from build123d import *

# Parameters (mm, degrees)
EXTRUDE_1_DEPTH          = 10
HOLE_WIZARD_M1_6_1_D     = 1.25
HOLE_WIZARD_M1_6_1_DEPTH = 4.95
HOLE_WIZARD_M1_6_1_TIP   = 0.375537887


with BuildPart() as part:
    # 草图2 → 凸台-拉伸1 (new body)
    with BuildSketch(Plane(origin=(0, 0, 0), x_dir=(1, 0, 0), z_dir=(0, 1, 0))):
        Polygon((7, 11), (-7, 11), (-7, 1), (-10, 1), (-10, 0), (-6, 0), (-6, 10), (6, 10), (6, 0), (10, 0), (10, 1), (7, 1), align=None)
    extrude(amount=EXTRUDE_1_DEPTH)

    # M1.6 螺纹孔1
    with Locations(Plane(origin=(0, 0, -1), x_dir=(-1, 0, 0), z_dir=(0, 0, -1))):
        with Locations((-8.5, 8), (8.5, 8), (8.5, 2), (-8.5, 2)):
            Hole(HOLE_WIZARD_M1_6_1_D / 2, depth=HOLE_WIZARD_M1_6_1_DEPTH)
            with Locations((0, 0, -(HOLE_WIZARD_M1_6_1_DEPTH + HOLE_WIZARD_M1_6_1_TIP / 2))):  # 118° drill point
                Cone(0, HOLE_WIZARD_M1_6_1_D / 2, HOLE_WIZARD_M1_6_1_TIP, mode=Mode.SUBTRACT)


solid = part.part
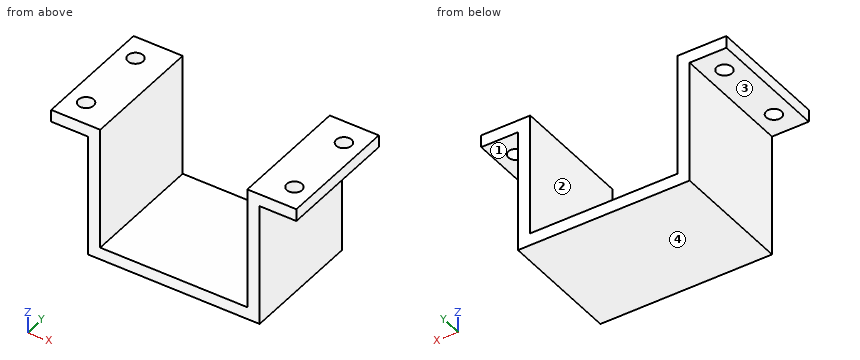
Read the model definition and answer for the solid it produces. Units are mm, in the model's axes. Face numbers are marked on the shaded views. A direction names the side the tool comes from. Round coordinates to 2 decimals unless told otherwise and drop trailing zeros. Write each loop counter-clockwise with the first axis right and the second up, starting at its lowest first coordinate (ties: lowest second). Pieces come first, ordered by that corner, then holes.
1. The part is cut by section C-C, the plane y = 8. Determine the outline of the cut face in (x, z) (3 decimals).
2. Straight lines are drawn through the part: L1, parallel to Y at x = 8.5, z = -0.65 (3 decimals); L2, parallel to X at y = 9, z = -8.75; L3, parallel to Z at x = -0.5, y = 9.25. For each, find the intervals that lie inside material, in ascending order.
3. Given pin 1 Ø5 at (y, z) = (5.5, -6) entering from -X; pin 2 Ø3 at (x, y) = (-1, 5) entering from +Z; pin 3 Ø3 at (y, z) = (3, -6.5) entering from +X, each flat-ended and moving along its own axis, determine where each tip first touches the part or whether it passes through.
4. The part is cut by section B-B, the plane x = -8.5. Determine the outline of the cut face in (y, z) (3 decimals).
5. The part is cut by section A-A, the plane z = -8.5. Determine the outline of the cut face in (x, y).
6. The part is cut by section D-D, the plane y = 6. Determine the outline of the cut face in (x, z).
7. Which of the six approach directions +Z, -Z, +X, -X, +Y, -Y give full straight-line access (tool end or side, diameter ignored) to the marked faces 1, 2, 3 and 4?
Values:
1. outline: (-10, -1) - (-9.125, -1) - (-9.125, 0) - (-10, 0) - close; (-7.875, -1) - (-7, -1) - (-7, -11) - (7, -11) - (7, -1) - (7.875, -1) - (7.875, 0) - (6, 0) - (6, -10) - (-6, -10) - (-6, 0) - (-7.875, 0) - close; (9.125, -1) - (10, -1) - (10, 0) - (9.125, 0) - close
2. L1: y = 0 to 1.375, 2.625 to 7.375, 8.625 to 10
2. L2: x = -7 to -6, 6 to 7
2. L3: z = -11 to -10
3. pin 1: stops at x = -7
3. pin 2: stops at z = -10
3. pin 3: stops at x = 7
4. outline: (0, -1) - (1.375, -1) - (1.375, 0) - (0, 0) - close; (2.625, -1) - (7.375, -1) - (7.375, 0) - (2.625, 0) - close; (8.625, -1) - (10, -1) - (10, 0) - (8.625, 0) - close
5. outline: (-7, 0) - (-6, 0) - (-6, 10) - (-7, 10) - close; (6, 0) - (7, 0) - (7, 10) - (6, 10) - close
6. outline: (-10, -1) - (-7, -1) - (-7, -11) - (7, -11) - (7, -1) - (10, -1) - (10, 0) - (6, 0) - (6, -10) - (-6, -10) - (-6, 0) - (-10, 0) - close
7. face 1: -Z, +X, +Y, -Y
7. face 2: +Z, +Y, -Y
7. face 3: -Z, -X, +Y, -Y
7. face 4: -Z, +X, -X, +Y, -Y
